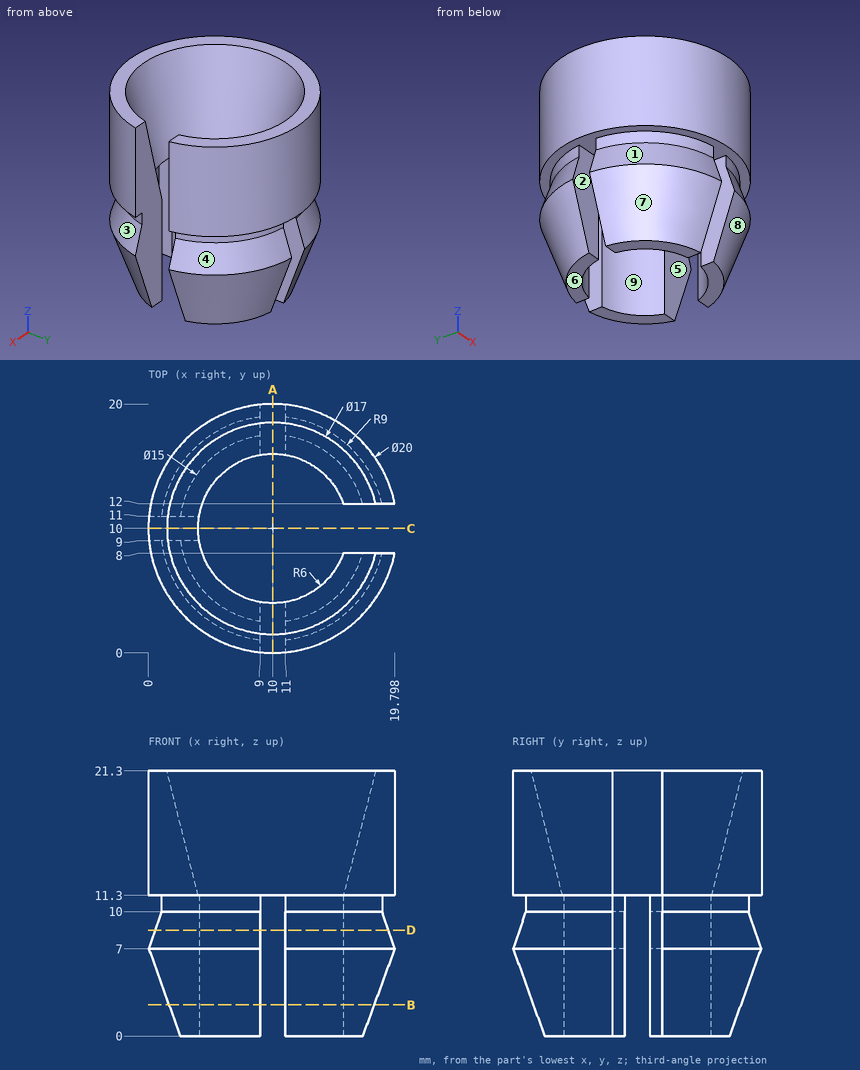
Part print with two shaded views. Sizes in mm from the minimum x, y, z corner. A direction names the side the tool comes from. Coordinates: 2 decimals unless noted, no trailing zeros. Order: outer loops, then holes, each group sorted by start corner. A loop starts at its lowest first (then second) coordinate and runs counter-clockwise, first axis right, second up.
(1) Saw through at C-C, the plane y = 10. Write the cut outline in (x, z).
Solution:
outline: (0, 11.3) - (4, 11.3) - (1.5, 21.3) - (0, 21.3) - close
(2) Saw through at D-D, the plane z = 8.5. Write the cut outline in (x, y).
Solution:
outline: (0.55, 9) arc R9.5 ccw to (9, 0.55) - (9, 4.08) arc R6 cw to (4.08, 9) - close; (0.55, 11) - (4.08, 11) arc R6 cw to (9, 15.92) - (9, 19.45) arc R9.5 ccw to start; (11, 0.55) arc R9.5 ccw to (19.29, 8) - (15.66, 8) arc R6 cw to (11, 4.08) - close; (11, 15.92) arc R6 cw to (15.66, 12) - (19.29, 12) arc R9.5 ccw to (11, 19.45) - close
(3) Which spindle directions (+Z, -Z, +X, -X, +Y, -Y) get a long thin tool onto all of the face, cutting with end or side? Do the marked faces 1, 2, 3, 4 and 5. Say none if no direction does.
Solution:
face 1: -X, -Y
face 2: -Z, +X, -X
face 3: +X, -Y
face 4: +X, +Y
face 5: +Z, -Z, +X
(4) Mould opens along X. For the marked faces 6, 7, 8 and 9 say: released by +X, released by -X, zero draft, split by the parting line, or undercut.
Solution:
face 6: zero draft
face 7: released by -X
face 8: released by +X
face 9: undercut
(5) Drill centre lines: L1, parallel to Y at x = 7.75, z = 6.75; L2, parallel to Y at x = 11.75, z = 12.25; L3, parallel to X at y = 6.75, z = 7.5. Where is each one in solid material? Low to high.
Solution:
L1: y = 0.35 to 4.44, 15.56 to 19.65
L2: y = 0.15 to 4.01, 15.99 to 19.85
L3: x = 0.72 to 4.96, 15.04 to 19.28
(6) Saw through at A-A, the plane x = 10. Write the cut outline in (y, z), and give its area (3 significant figures).
Solution:
outline: (0, 11.3) - (4, 11.3) - (1.5, 21.3) - (0, 21.3) - close; (16, 11.3) - (20, 11.3) - (20, 21.3) - (18.5, 21.3) - close
area: 55.0 mm2
(7) Pin check, flat tips, straight feed: pin 1 Ø2 at (x, z) = (3, 3) entering from +Y; pin 2 Ø1.2 at (x, z) = (17.5, 14) entering from +Y; pin 3 Ø1 at (y, z) = (16, 8) entering from +X. Stop position of each tip, or through.
Solution:
pin 1: stops at y = 16.24
pin 2: stops at y = 17.24
pin 3: stops at x = 18
(8) Saw through at B-B, the plane z = 2.5. Write the cut outline in (x, y).
Solution:
outline: (1.67, 9) arc R8.39 ccw to (9, 1.67) - (9, 4.08) arc R6 cw to (4.08, 9) - close; (1.67, 11) - (4.08, 11) arc R6 cw to (9, 15.92) - (9, 18.33) arc R8.39 ccw to start; (11, 1.67) arc R8.39 ccw to (18.15, 8) - (15.66, 8) arc R6 cw to (11, 4.08) - close; (11, 15.92) arc R6 cw to (15.66, 12) - (18.15, 12) arc R8.39 ccw to (11, 18.33) - close
